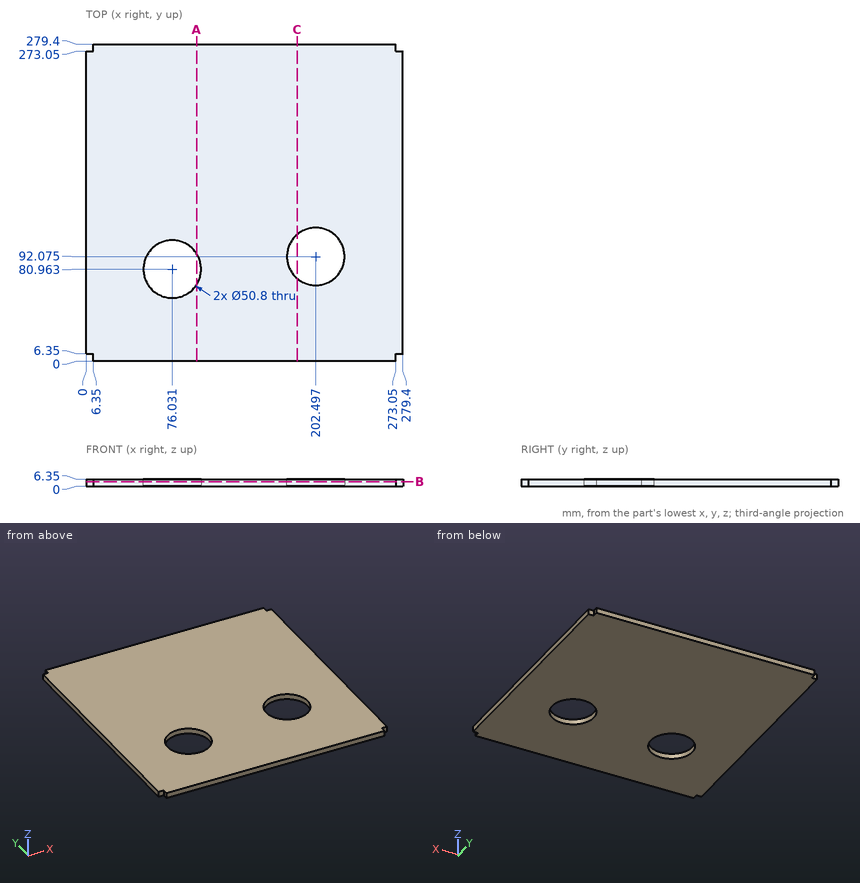
Check sheet for the drawn part. Datum: minimum x, y, z corner. Units: mm. Coordinates: 2 decimals unless noted, no trailing zeros. Loops run counter-clockwise (first coordinate to the right, second up) from the corner with the lowest first, then second, coordinate; pieces in that order, holes last. Notation, with made-up numbers: (76, -3) - (120, -3) arc R22 cw to (120, 13) - close; hole circle Ø3 at (36.5, 29.5). An arc over 180 degrees is marked (long way). Put each result on its own line as item: value.
Item 1: Gauge pin test, flat ends, axial feed: pin 1 Ø1.9 at (y, z) = (4, 3.5) entering from +X; pin 2 Ø3 at (x, z) = (276, 4) entering from -Y. Record the tip position at first contact, or that the pin passes through.
Conclusion:
pin 1: stops at x = 273.05
pin 2: stops at y = 6.35
Item 2: Section check B-B (z = 4). Give the number of separate pieces and of enclosed holes in the cut face, then the cut area to 4 significant figures.
Conclusion:
separate pieces: 1
enclosed holes: 2
area: 73,850 mm2
Item 3: Scan lines: line 1 along X through (y, z) = (79.5, 6.25) (1 decimal); line 2 along Y through (x, z) = (74.5, 3.25); line 3 along Y through (x, z) = (61, 5) (1 decimal). Record each from-to range of solid material in increasing order.
Conclusion:
line 1: x = 0 to 50.7, 101.4 to 180.4, 224.6 to 279.4
line 2: y = 0 to 55.61, 106.32 to 279.4
line 3: y = 0 to 60.5, 101.4 to 279.4
Item 4: Section check A-A (x = 97.5). Enter the section's corners in (y, z), then the cut area to 3 significant figures.
Conclusion:
outline: (0, 0) - (67.39, 0) - (67.39, 6.35) - (0, 6.35) - close; (94.54, 0) - (279.4, 0) - (279.4, 6.35) - (94.54, 6.35) - close
area: 1,600 mm2
Item 5: Section check C-C (x = 186). Enter the section's corners in (y, z), then the cut area to 3 significant figures.
Conclusion:
outline: (0, 0) - (72.76, 0) - (72.76, 6.35) - (0, 6.35) - close; (111.39, 0) - (279.4, 0) - (279.4, 6.35) - (111.39, 6.35) - close
area: 1,530 mm2
